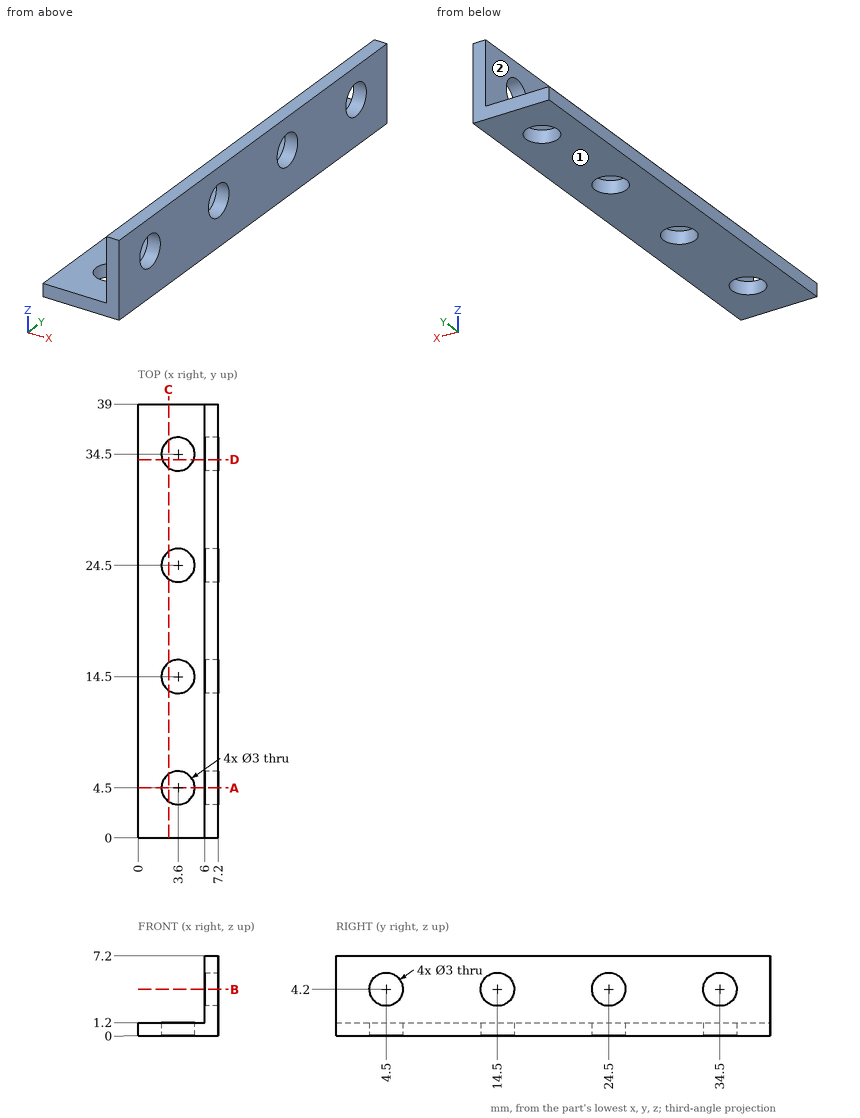
For this review, use the dimensioned drawing (mm, ordinates from the lowest corner) and the shaded views. A direction names the side the tool comes from. Give positions to 0.01 mm unless a question says otherwise; leave off trailing zeros. Write each loop counter-clockwise with the first axis right and the second up, starting at its lowest first coordinate (ties: lowest second). Pieces come first, ordered by that corner, then holes.
(1) To check wall thickness, follow L1, parallel to Y at x = 3.6, z = 0.5; L2, parallel to X at y = 4, z = 2; L3, parallel to Z at x = 4, y = 27. State the ranges of each line that lie inside material, in increasing order.
(2) Consider section D-D, the plane y = 34. Give the boundary of the cut face in (x, z), and give its area (3 significant figures).
(3) Tool access review of the marked faces 1 and 2: name each direction out of +Z, -Z, +X, -X, +Y, -Y from which nothing blocks a thin tool from reaching the whole face with its end or side.
(4) Consider section A-A, the plane y = 4.5. Give the boundary of the cut face in (x, z), and give its area (3 significant figures).
(5) Consider section C-C, the plane x = 2.75. Give the boundary of the cut face in (y, z), and give its area (3 significant figures).
(6) Consider section B-B, the plane z = 4.2. Give the boundary of the cut face in (x, y).
(7) For P1, Ø4, axis at y = 34.5, z = 4.2, coming from the -X side, flat-tipped, find the tip position at first contact; note if it passes through.
Returned:
1. L1: y = 0 to 3, 6 to 13, 16 to 23, 26 to 33, 36 to 39
1. L2: x = 6 to 7.2
1. L3: z = 0 to 1.2
2. outline: (0, 0) - (2.19, 0) - (2.19, 1.2) - (0, 1.2) - close; (5.01, 0) - (7.2, 0) - (7.2, 2.79) - (6, 2.79) - (6, 1.2) - (5.01, 1.2) - close; (6, 5.61) - (7.2, 5.61) - (7.2, 7.2) - (6, 7.2) - close
2. area: 9.05 mm2
3. face 1: -Z, +X, -X, +Y, -Y
3. face 2: +Z, -X, +Y, -Y
4. outline: (0, 0) - (2.1, 0) - (2.1, 1.2) - (0, 1.2) - close; (5.1, 0) - (7.2, 0) - (7.2, 2.7) - (6, 2.7) - (6, 1.2) - (5.1, 1.2) - close; (6, 5.7) - (7.2, 5.7) - (7.2, 7.2) - (6, 7.2) - close
4. area: 8.64 mm2
5. outline: (0, 0) - (3.26, 0) - (3.26, 1.2) - (0, 1.2) - close; (5.74, 0) - (13.26, 0) - (13.26, 1.2) - (5.74, 1.2) - close; (15.74, 0) - (23.26, 0) - (23.26, 1.2) - (15.74, 1.2) - close; (25.74, 0) - (33.26, 0) - (33.26, 1.2) - (25.74, 1.2) - close; (35.74, 0) - (39, 0) - (39, 1.2) - (35.74, 1.2) - close
5. area: 34.9 mm2
6. outline: (6, 0) - (7.2, 0) - (7.2, 3) - (6, 3) - close; (6, 6) - (7.2, 6) - (7.2, 13) - (6, 13) - close; (6, 16) - (7.2, 16) - (7.2, 23) - (6, 23) - close; (6, 26) - (7.2, 26) - (7.2, 33) - (6, 33) - close; (6, 36) - (7.2, 36) - (7.2, 39) - (6, 39) - close
7. P1: stops at x = 6
